Work out the finished part from the listing and answer in its coordinate system (mm). A direction names the side the tool comes from. Give positions to 0.01 mm unless a question says otherwise; leave off trailing zeros. Loops run counter-clockwise (first coordinate to the right, second up) from the corner with the lowest first, then second, coordinate; pieces in that order, holes last. Notation, with made-up numbers: (36.25, -8) - (40.25, -8) arc R8 cw to (40.25, 0) - close; hole circle Ø6 at (72.5, -8.5). An arc over 180 degrees is marked (long way). Use one line per item in the form item = value. Start each with the question number.
from build123d import *

# Parameters (mm, degrees)
SKETCH1_W           = 32.1
SKETCH1_H           = 32.1
SKETCH1_R           = 0.95
BOSS_EXTRUDE1_DEPTH = 1.65
SKETCH2_W           = 22.1
SKETCH2_H           = 6.75
BOSS_EXTRUDE2_DEPTH = 2.5
SKETCH3_R           = 0.625
BOSS_EXTRUDE3_DEPTH = 5
SKETCH4_R           = 7
BOSS_EXTRUDE4_DEPTH = 17
FILLET1_R           = 2


with BuildPart() as part:
    # Sketch1 → Boss-Extrude1 (new body)
    with BuildSketch(Plane(origin=(0, 0, 0), x_dir=(1, 0, 0), z_dir=(0, 1, 0))):
        Rectangle(SKETCH1_W, SKETCH1_H)
        with Locations(Location((-14.05, 14.05, 0), (0, 0, 270))):
            Circle(SKETCH1_R, mode=Mode.SUBTRACT)
        with Locations(Location((14.05, 14.05, 0), (0, 0, 90))):
            Circle(SKETCH1_R, mode=Mode.SUBTRACT)
        with Locations(Location((14.05, -14.05, 0), (0, 0, 270))):
            Circle(SKETCH1_R, mode=Mode.SUBTRACT)
        with Locations(Location((-14.05, -14.05, 0), (0, 0, 90))):
            Circle(SKETCH1_R, mode=Mode.SUBTRACT)
    extrude(amount=BOSS_EXTRUDE1_DEPTH)

    # Sketch2 → Boss-Extrude2 (add)
    with BuildSketch(Plane.XZ):
        with Locations((0, 12.675)):
            Rectangle(SKETCH2_W, SKETCH2_H)
    extrude(amount=BOSS_EXTRUDE2_DEPTH)

    # Sketch3 → Boss-Extrude3 (add)
    with BuildSketch(Plane(origin=(0, 1.65, 0), x_dir=(1, 0, 0), z_dir=(0, 1, 0))):
        with BuildLine():
            Line((9.9, 2.25), (8.55, 2.25))
            Line((8.55, 2.25), (8.55, 8.55))
            Line((8.55, 8.55), (-8.55, 8.55))
            Line((-8.55, 8.55), (-8.55, 2.25))
            Line((-8.55, 2.25), (-9.9, 2.25))
            ThreePointArc((-9.9, 2.25), (-12.15, 0), (-9.9, -2.25))
            Line((-9.9, -2.25), (-8.55, -2.25))
            Line((-8.55, -2.25), (-8.55, -8.55))
            Line((-8.55, -8.55), (8.55, -8.55))
            Line((8.55, -8.55), (8.55, -2.25))
            Line((8.55, -2.25), (9.9, -2.25))
            ThreePointArc((9.9, -2.25), (12.15, 0), (9.9, 2.25))
        make_face()
        with Locations(Location((9.9, 0, 0), (0, 0, 270))):
            Circle(SKETCH3_R, mode=Mode.SUBTRACT)
        with Locations(Location((-9.9, 0, 0), (0, 0, 90))):
            Circle(SKETCH3_R, mode=Mode.SUBTRACT)
    extrude(amount=BOSS_EXTRUDE3_DEPTH)

    # Sketch4 → Boss-Extrude4 (add)
    with BuildSketch(Plane(origin=(0, 6.65, 0), x_dir=(1, 0, 0), z_dir=(0, 1, 0))):
        with Locations(Location((0, 0, 0), (0, 0, 270))):
            Circle(SKETCH4_R)
    extrude(amount=BOSS_EXTRUDE4_DEPTH)

    # Fillet1
    fillet1_edges = [part.edges().sort_by_distance(p)[0] for p in [
        (-16.05, 0.825, -16.05),
        (16.05, 0.825, -16.05),
        (16.05, 0.825, 16.05),
        (-16.05, 0.825, 16.05),
    ]]
    fillet(fillet1_edges, radius=FILLET1_R)


solid = part.part
1) Determine the mould class of faces 4 (the flat face through (9, 4, 2.25)), 5 (the cylindrical face through (-13.21, 0.81, 13.61)), 6 (the cylindrical face through (15.45, 0.84, -15.48)) for opening direction X: released by +X, released by -X, zero draft, split by the parting line, or undercut.
2) Flat-ended cylindrical pins translate along their axes: pin 1 Ø5 at (y, z) = (6, -0.5) entering from -X; pin 2 Ø4 at (x, y) = (1.5, 4.5) entering from -Z; pin 3 Ø2 at (y, z) = (3, -8.5) entering from +X. Find the tip coordinate at first contact, or state that the pin passes through.
3) A tool of negligible diameter and unlimited length cuts with its end or side. For faces 1 (the flat face through (10, 1.65, 0)), 2 (the flat face through (-11.05, -1, 13)), 3 (the flat face through (0, -1, 9.3)), from which of +Z, -Z, +X, -X, +Y, -Y can it reach the whole face along a straight path? Write none if from no direction.
4) A cutting plane is placed at A-A (z = 11.5). Give the vertices of the cut face in (x, y).
5) Find the intervals of material crossed by probe 1 along X at (y, z) = (0.9, 14.05); probe 2 along Z at (x, y) = (-9.9, 4.95) (3 decimals); probe 3 along Y at (x, z) = (-0.5, 13), in increasing order.
6) A cutting plane is placed at D-D (x = -5). Give the vertices of the cut face in (y, z), plus the area to 3 significant figures.
7) A cutting plane is placed at B-B (x = 0). Give the vertices of the cut face in (y, z), plus the area to 3 significant figures.
8) A cutting plane is placed at C-C (y = 15.25). Give the vertices of the cut face in (x, z).
Answer sheet:
q1.face_4 = zero draft
q1.face_5 = undercut
q1.face_6 = released by +X
q2.pin_1 = -12.15
q2.pin_2 = -8.55
q2.pin_3 = 8.55
q3.face_1 = +Y
q3.face_2 = +Z, -Z, -X, -Y
q3.face_3 = -Z, +X, -X, -Y
q4.outline = (-16.05, 0) - (-11.05, 0) - (-11.05, -2.5) - (11.05, -2.5) - (11.05, 0) - (16.05, 0) - (16.05, 1.65) - (-16.05, 1.65) - close
q5.probe_1 = -16.05 to -15, -13.1 to 13.1, 15 to 16.05
q5.probe_2 = -2.25 to -0.625, 0.625 to 2.25
q5.probe_3 = -2.5 to 1.65
q6.outline = (-2.5, 9.3) - (0, 9.3) - (0, -16.05) - (1.65, -16.05) - (1.65, -8.55) - (6.65, -8.55) - (6.65, -4.9) - (23.65, -4.9) - (23.65, 4.9) - (6.65, 4.9) - (6.65, 8.55) - (1.65, 8.55) - (1.65, 16.05) - (-2.5, 16.05) - close
q6.area = 322 mm²
q7.outline = (-2.5, 9.3) - (0, 9.3) - (0, -16.05) - (1.65, -16.05) - (1.65, -8.55) - (6.65, -8.55) - (6.65, -7) - (23.65, -7) - (23.65, 7) - (6.65, 7) - (6.65, 8.55) - (1.65, 8.55) - (1.65, 16.05) - (-2.5, 16.05) - close
q7.area = 393 mm²
q8.outline = circle Ø14 at (0, 0)
